Source: CAD feature listing. Evaluate the final solid. Frame: model axes, mm. Face numbers are marked on the shaded views. A direction names the side the tool comes from. Give positions to 0.01 mm unless a question says otherwise; leave off trailing zeros. Order: outer loops, then holes, each group sorted by start corner. A loop starts at its lowest first (then second) coordinate and runs counter-clockwise, first axis right, second up. Notation, with made-up numbers: M 20,89.25 L 75,89.25 A27 cw 75,121.25 Z; hole C 31.25,-17.75 d4. An arc over 180 degrees is marked long. Use CSV: the item, a comma, the result in double quotes. Start each with the question number.
1. Section query D-D, the plane y = -7.75. State how many separate pieces and enclosed holes the cut face has, plus the area to 3 significant figures.
2. Line query: line 1 along Z through (x, y) = (0, -7.25); line 2 along Y through (x, z) = (2.5, -10); line 3 along Z through (x, y) = (-9, -2.5). Output: solid intervals per line, ascending. Write a range as [from, to].
3. Section query A-A, the plane z = 0. Return the cut outline in (x, y).
4. Pin query (flat end, axial travel): P1, Ø4, axis at y = -15, z = -3.5, coming from the -X side; P2, Ø6, axis at x = 1.5, z = 11.5, coming from the +Y side; P3, Ø0.5, axis at y = -12.5, z = -2, coming from the +X side; P4, Ø4, axis at y = 0, z = 14, coming from the -X side. Return the tip coordinate at first contact, or that it passes through.
5. Reachability of the marked faces 1, 2, 3, 4 and 5 from +Z, -Z, +X, -X, +Y, -Y: full face, straight path, thin tool, end or side. Return the list, or none.
6. Section query C-C, the plane y = -12.25. Return the cut outline in (x, z), plus the area to 3 significant figures.
7. Mould query, pull axis X, two halves, no side actions, for the marked faces 6, 7 and 8. Classes: released by +X, released by -X, zero draft, split by the parting line, or undercut.
8. Section query B-B, the plane y = -17.5. Return the cut outline in (x, z).
from build123d import *
from build123d.topology import SkipClean

# Parameters (mm, degrees)
FEET_DEPTH            = 4.572
SWITCH_HOLE_REACH     = 31.195
SKETCH2_W             = 12.954
SKETCH2_H             = 12.065
SQUARE_DEPTH          = 31.164446025
SQUARE_DEPTH_BACK     = 31.164446025
SKETCH6_W             = 5.461
SKETCH6_H             = 5.842
EXTRUDE3_START        = -0.508
SKETCH4_W             = 12.954
SKETCH4_H             = 12.065
EXTRUDE3_DEPTH        = 0.508
SKETCH5_W             = 15.621
SKETCH5_H             = 12.065
SWITCH_HOLE2_DEPTH    = 1.524
TAB_CIRC_CUTOUT_DEPTH = 17.066
TAB_START             = -6
TAB_TOP_OUTLINE_W     = 2.54
TAB_TOP_OUTLINE_H     = 1.905
TAB_TOP_DEPTH         = 6
TAB_WEDGE_DEPTH       = 3
SKETCH11_W            = 4.476
SKETCH11_H            = 10.247840718
CUT_TAB_DEPTH         = 3.556
FILLET1_R             = 0.762


# Read off the part's stored shape, not the designer's step: tab circ cutout, tab top
with BuildPart() as part:
    # Sketch1 → Revolve1 (revolve)
    with BuildSketch(Plane.XY, mode=Mode.PRIVATE) as revolve1_sk:
        with BuildLine():
            Line((14.732, 0), (16.51, 0))
            ThreePointArc((16.51, 0), (15.124670081, 2.159981002), (12.7, 3))
            Line((12.7, 3), (12.7, -11.224))
            Line((12.7, -11.224), (0, -11.224))
            Line((0, -11.224), (0, -14.526))
            Line((0, -14.526), (8.6995, -14.526))
            Line((8.6995, -14.526), (8.6995, -19.098))
            Line((8.6995, -19.098), (14.732, -19.098))
            Line((14.732, -19.098), (14.732, 0))
        make_face()
    revolve(revolve1_sk.sketch.rotate(Axis((0, 3, 0), (0, -1, 0)), 180), axis=Axis((0, 3, 0), (0, -1, 0)))

    # Sketch3 → feet (cut)
    with BuildSketch(Plane.XZ.offset(19.098)):
        with BuildLine():
            ThreePointArc((-7.2136, 12.845069055), (-14.732, 0), (-7.2136, -12.845069055))
            Line((-7.2136, -12.845069055), (-4.259755172, -7.585234744))
            ThreePointArc((-4.259755172, -7.585234744), (-8.6995, 0), (-4.259755172, 7.585234744))
            Line((-4.259755172, 7.585234744), (-7.2136, 12.845069055))
        make_face()
        with BuildLine():
            Line((4.259755172, -7.585234744), (7.2136, -12.845069055))
            ThreePointArc((7.2136, -12.845069055), (14.732, 0), (7.2136, 12.845069055))
            Line((7.2136, 12.845069055), (4.259755172, 7.585234744))
            ThreePointArc((4.259755172, 7.585234744), (8.6995, 0), (4.259755172, -7.585234744))
        make_face()
    extrude(amount=-FEET_DEPTH, mode=Mode.SUBTRACT)

    # Sketch2 → switch hole (cut, up to next)
    with BuildSketch(Plane.XZ.offset(14.526), mode=Mode.PRIVATE) as switch_hole_sk1:
        Rectangle(SKETCH2_W, SKETCH2_H)
    switch_hole_tool1 = extrude(switch_hole_sk1.sketch, amount=-SWITCH_HOLE_REACH, mode=Mode.PRIVATE) & part.part
    add(switch_hole_tool1.solids().sort_by_distance((0, -14.526, 0))[0], mode=Mode.SUBTRACT)

    # Sketch6 → square (cut, two sides: drawn at the far end of the back side and taken through both)
    with BuildSketch(Plane(origin=(0, 0, 0), x_dir=(0, 0, -1), z_dir=(1, 0, 0)).offset(-SQUARE_DEPTH_BACK)):
        with Locations((0, -8.303)):
            Rectangle(SKETCH6_W, SKETCH6_H)
    extrude(amount=SQUARE_DEPTH + SQUARE_DEPTH_BACK, mode=Mode.SUBTRACT)

    # Sketch4 → Extrude3 (cut)
    with BuildSketch(Plane(origin=(0, -11.224, 0), x_dir=(1, 0, 0), z_dir=(0, 1, 0)).offset(EXTRUDE3_START)):
        with BuildLine():
            Line((11.099066166, -2.7305), (12.402998418, -2.7305))
            ThreePointArc((12.402998418, -2.7305), (12.7, 0), (12.402998418, 2.7305))
            Line((12.402998418, 2.7305), (11.099066166, 2.7305))
            ThreePointArc((11.099066166, 2.7305), (0, 11.43), (-11.099066166, 2.7305))
            Line((-11.099066166, 2.7305), (-12.402998418, 2.7305))
            ThreePointArc((-12.402998418, 2.7305), (-12.7, 0), (-12.402998418, -2.7305))
            Line((-12.402998418, -2.7305), (-11.099066166, -2.7305))
            ThreePointArc((-11.099066166, -2.7305), (0, -11.43), (11.099066166, -2.7305))
        make_face()
        Rectangle(SKETCH4_W, SKETCH4_H, mode=Mode.SUBTRACT)
    extrude(amount=EXTRUDE3_DEPTH, mode=Mode.SUBTRACT)

    # Sketch5 → switch hole2 (cut)
    with BuildSketch(Plane(origin=(0, -11.732, 0), x_dir=(1, 0, 0), z_dir=(0, 1, 0))):
        Rectangle(SKETCH5_W, SKETCH5_H)
    extrude(amount=-SWITCH_HOLE2_DEPTH, mode=Mode.SUBTRACT)

    # tab circ cutout outline → tab circ cutout (cut)
    with BuildSketch(Plane.XZ):
        with BuildLine():
            ThreePointArc((-4.5, 9.109094357), (0, 10.16), (4.5, 9.109094357))
            Line((4.5, 9.109094357), (4.5, 14.027894496))
            ThreePointArc((4.5, 14.027894496), (0, 14.732), (-4.5, 14.027894496))
            Line((-4.5, 14.027894496), (-4.5, 9.109094357))
        make_face()
        with BuildLine():
            ThreePointArc((3, 12.340583455), (0, 12.7), (-3, 12.340583455))
            Line((-3, 12.340583455), (-3, 13.904034522))
            ThreePointArc((-3, 13.904034522), (0, 14.224), (3, 13.904034522))
            Line((3, 13.904034522), (3, 12.340583455))
        make_face(mode=Mode.SUBTRACT)
    tab_circ_cutout = extrude(amount=TAB_CIRC_CUTOUT_DEPTH, mode=Mode.SUBTRACT)

    # tab top outline → tab top (cut)
    with SkipClean():  # the faces are left unmerged after this step: merging them gives an invalid solid
        with BuildSketch(Plane(origin=(3, 0, 0), x_dir=(0, 0, -1), z_dir=(1, 0, 0)).offset(TAB_START)):
            with Locations((-13.610583455, -0.9525)):
                Rectangle(TAB_TOP_OUTLINE_W, TAB_TOP_OUTLINE_H)
        tab_top = extrude(amount=TAB_TOP_DEPTH, mode=Mode.SUBTRACT)
    add(part.part.scale(1), mode=Mode.REPLACE)  # the faces are merged on a copy

    # Sketch10 → tab wedge (add, symmetric)
    with BuildSketch(Plane(origin=(0, 0, 0), x_dir=(0, 0, -1), z_dir=(1, 0, 0))):
        Polygon((-13.904034522, -1.905), (-13.904034522, -14.478), (-17.651091727, -3.468159282), (-17.270091727, -3.468159282), (-17.270091727, -2.879362986), (-16.889091727, -2.879362986), (-16.889091727, -2.290566689), (-16.508091727, -2.290566689), (-16.508091727, -1.905), align=None)
    tab_wedge = extrude(amount=TAB_WEDGE_DEPTH, both=True)

    # Sketch11 → cut tab (cut)
    with BuildSketch(Plane.XY.offset(17.778091727)):
        with Locations((0, -9.354079641)):
            Rectangle(SKETCH11_W, SKETCH11_H)
    cut_tab = extrude(amount=-CUT_TAB_DEPTH, mode=Mode.SUBTRACT)

    # tab mirror: tab circ cutout, tab top, tab wedge, cut tab across plane
    add(tab_circ_cutout.mirror(Plane.XY), mode=Mode.SUBTRACT)
    add(tab_top.mirror(Plane.XY), mode=Mode.SUBTRACT)
    add(tab_wedge.mirror(Plane.XY))
    add(cut_tab.mirror(Plane.XY), mode=Mode.SUBTRACT)

    # Fillet1
    fillet1_edges = [part.edges().sort_by_distance(p)[0] for p in [
        (0, -19.098, -14.732),
        (14.732, -14.526, 0),
        (0, -19.098, 14.732),
        (-12.714216043, -14.526, -7.441809887),
    ]]
    fillet(fillet1_edges, radius=FILLET1_R)


solid = part.part
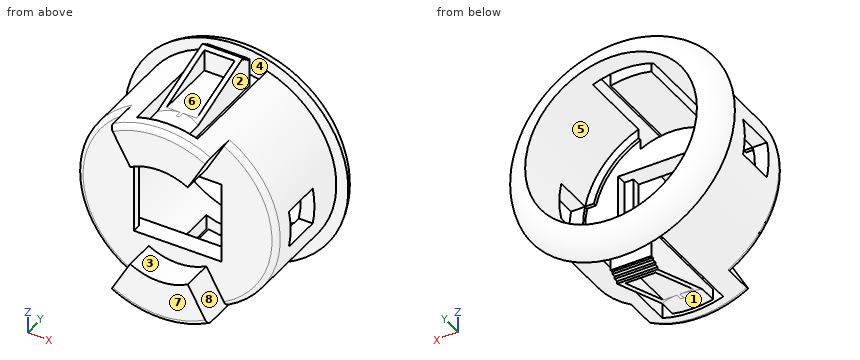
Result set:
1,separate pieces,"6"
1,enclosed holes,"0"
1,area,"141 mm2"
2,line 1,"[-14.22, -12.7], [12.7, 14.22]"
2,line 2,"[-19.1, -17.07]"
2,line 3,"[-11.66, -8.96], [8.96, 11.66]"
3,outline,"M -16.51,0 L -14.73,0 L -14.73,-5.38 L -12.7,-5.38 L -12.7,3 A3.92 ccw Z; M -14.73,-13.76 A0.76 ccw -13.97,-14.53 L -6.48,-14.53 L -6.48,-13.26 L -7.81,-13.26 L -7.81,-11.73 L -12.7,-11.73 L -12.7,-11.22 L -14.73,-11.22 Z; M 6.48,-14.53 L 13.97,-14.53 A0.76 ccw 14.73,-13.76 L 14.73,-11.22 L 12.7,-11.22 L 12.7,-11.73 L 7.81,-11.73 L 7.81,-13.26 L 6.48,-13.26 Z; M 12.7,-5.38 L 14.73,-5.38 L 14.73,0 L 16.51,0 A3.92 ccw 12.7,3 Z"
4,P1,"x = -14.61"
4,P2,"y = 3"
4,P3,"x = 14.63"
4,P4,"x = -11.34"
5,face 1,"-Z"
5,face 2,"+Z"
5,face 3,"-Y"
5,face 4,"none"
5,face 5,"+Y"
6,outline,"M -4.5,-14.03 L -4.5,-9.11 A10.16 ccw 4.5,-9.11 L 4.5,-14.03 A14.73 ccw 4.5,14.03 L 4.5,9.11 A10.16 ccw -4.5,9.11 L -4.5,14.03 A14.73 ccw Z; M -3,-14.66 L -2.24,-14.66 L -2.24,-14.22 L 2.24,-14.22 L 2.24,-14.66 L 3,-14.66 L 3,-12.34 A12.7 cw -3,-12.34 Z; M -3,12.34 A12.7 cw 3,12.34 L 3,14.66 L 2.24,14.66 L 2.24,14.22 L -2.24,14.22 L -2.24,14.66 L -3,14.66 Z; hole M -7.81,-6.03 L 7.81,-6.03 L 7.81,6.03 L -7.81,6.03 Z"
6,area,"430 mm2"
7,face 6,"undercut"
7,face 7,"zero draft"
7,face 8,"released by +X"
8,outline,"M -7.21,-12.85 A14.73 ccw 7.21,-12.85 L 4.26,-7.59 A8.7 cw -4.26,-7.59 Z; M -7.21,12.85 L -4.26,7.59 A8.7 cw 4.26,7.59 L 7.21,12.85 A14.73 ccw Z"
